Can you work these out from the model? Positions are in its coordinate system, mm. A direction names the side the tool comes from. Coordinates: 2 decimals unless noted, no trailing zeros. Write each loop counter-clockwise with the first axis right and the second up, starting at its lowest first coordinate (ties: lowest second). Pieces come first, ordered by that corner, then holes.
```python
from build123d import *

# Parameters (mm, degrees)
SKETCH1_R           = 10
BOSS_EXTRUDE1_DEPTH = 3
SKETCH1_6_R         = 1.5
CUT_EXTRUDE2_DEPTH  = 4
SKETCH1_7_R         = 1.5
CUT_EXTRUDE3_DEPTH  = 4
SKETCH3_R           = 2.5
CUT_EXTRUDE5_DEPTH  = 2


with BuildPart() as part:
    # Sketch1 → Boss-Extrude1 (new body)
    with BuildSketch(Plane.XY):
        Circle(SKETCH1_R)
    extrude(amount=BOSS_EXTRUDE1_DEPTH)

    # Sketch1<6> → Cut-Extrude2 (cut, through all)
    with BuildSketch(Plane.XY):
        Circle(SKETCH1_6_R)
    extrude(amount=CUT_EXTRUDE2_DEPTH, mode=Mode.SUBTRACT)

    # Sketch1<7> → Cut-Extrude3 (cut, through all)
    with BuildSketch(Plane.XY):
        with Locations((0, -7)):
            Circle(SKETCH1_7_R)
        with Locations((-4.114496766, -5.663118961)):
            Circle(SKETCH1_7_R)
        with Locations((-6.657395614, -2.163118961)):
            Circle(SKETCH1_7_R)
        with Locations((-6.657395614, 2.163118961)):
            Circle(SKETCH1_7_R)
        with Locations((-4.114496766, 5.663118961)):
            Circle(SKETCH1_7_R)
        with Locations((0, 7)):
            Circle(SKETCH1_7_R)
        with Locations((4.114496766, 5.663118961)):
            Circle(SKETCH1_7_R)
        with Locations((6.657395614, 2.163118961)):
            Circle(SKETCH1_7_R)
        with Locations((6.657395614, -2.163118961)):
            Circle(SKETCH1_7_R)
        with Locations((4.114496766, -5.663118961)):
            Circle(SKETCH1_7_R)
    extrude(amount=CUT_EXTRUDE3_DEPTH, mode=Mode.SUBTRACT)

    # Sketch3 → Cut-Extrude5 (cut)
    with BuildSketch(Plane.XY.offset(3)):
        Circle(SKETCH3_R)
    extrude(amount=-CUT_EXTRUDE5_DEPTH, mode=Mode.SUBTRACT)


solid = part.part
```
1. If we section it at D-D, the plane y = -4.75: List the corners of the cut face in (x, z) for me, plus the area to 3 significant figures.
2. If I drill on L1, parallel to Y at x = 0, z = 1.1; L2, parallel to Y at x = 4.25, z = 1.05; L3, parallel to X at y = -2.25, z = 0.3, over which ranges is the centre line in solid material (lowest first)?
3. Which directions (+Z, -Z, +X, -X, +Y, -Y) give clear straight access to the entire face, cutting with the end or side of a thin tool? Please do faces 4 (the face through (-0.54, -2.44, 2.01)), 5 (the face through (0, -2, 0)).
4. If we section it at B-B, the plane x = 3.25: List the corners of the cut face in (y, z) for me.
5. If we section it at A-A, the plane y = 0: List the corners of the cut face in (x, z) for me, plus the area to 3 significant figures.
6. We'd pull the mould along X, two halves only. Please class faces 1 (the face through (-2.684, -5.213, 1.479)), 2 (the face through (2, -2, 3)), 3 (the face through (-2.17, -9.76, 1.48)): released by +X, released by -X, zero draft, split by the parting line, or undercut.
7. I'm going to push flat-ended pins straight in: P1, Ø1.8, axis at x = 0, y = 7, coming from the +Z side; P2, Ø1.5, axis at y = 8, z = 1.5, coming from the +X side; P3, Ø1, axis at y = 5, z = 2.5, coming from the +X side; P4, Ø1.5, axis at x = -0.5, y = 1, coming from the +Z side. Where does each tip first touch, or does it pass through?
8. If we section it at C-C, the plane x = 0: List the corners of the cut face in (y, z) for me, plus the area to 3 significant figures.
Answers:
1. outline: (-8.8, 0) - (-5.3, 0) - (-5.3, 3) - (-8.8, 3) - close; (-2.92, 0) - (2.92, 0) - (2.92, 3) - (-2.92, 3) - close; (5.3, 0) - (8.8, 0) - (8.8, 3) - (5.3, 3) - close
1. area: 38.5 mm2
2. L1: y = -10 to -8.5, -5.5 to -2.5, 2.5 to 5.5, 8.5 to 10
2. L2: y = -9.05 to -7.16, -4.17 to 4.17, 7.16 to 9.05
2. L3: x = -9.74 to -8.15, -5.16 to 5.16, 8.15 to 9.74
3. face 4: +Z
3. face 5: -Z, +X, -X, +Y, -Y
4. outline: (-9.46, 0) - (-6.89, 0) - (-6.89, 3) - (-9.46, 3) - close; (-4.44, 0) - (4.44, 0) - (4.44, 3) - (-4.44, 3) - close; (6.89, 0) - (9.46, 0) - (9.46, 3) - (6.89, 3) - close
5. outline: (-10, 0) - (-1.5, 0) - (-1.5, 1) - (-2.5, 1) - (-2.5, 3) - (-10, 3) - close; (1.5, 0) - (10, 0) - (10, 3) - (2.5, 3) - (2.5, 1) - (1.5, 1) - close
5. area: 47.0 mm2
6. face 1: undercut
6. face 2: zero draft
6. face 3: split by the parting line
7. P1: passes through
7. P2: stops at x = 6.89
7. P3: stops at x = 8.93
7. P4: stops at z = 1
8. outline: (-10, 0) - (-8.5, 0) - (-8.5, 3) - (-10, 3) - close; (-5.5, 0) - (-1.5, 0) - (-1.5, 1) - (-2.5, 1) - (-2.5, 3) - (-5.5, 3) - close; (1.5, 0) - (5.5, 0) - (5.5, 3) - (2.5, 3) - (2.5, 1) - (1.5, 1) - close; (8.5, 0) - (10, 0) - (10, 3) - (8.5, 3) - close
8. area: 29.0 mm2
